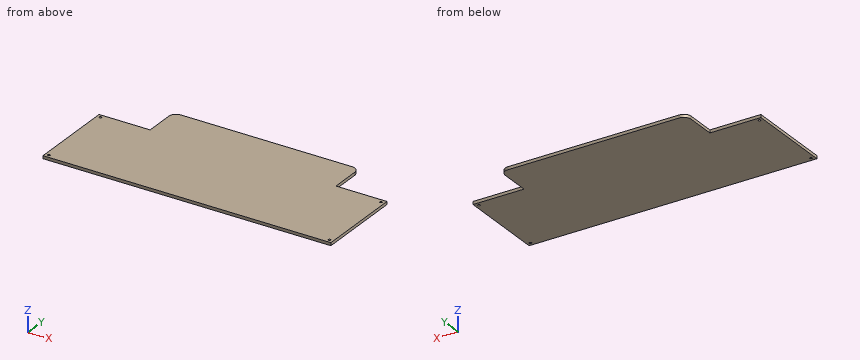
from build123d import *

# Parameters (mm, degrees)
SKETCH_1_R      = 1.6
EXTRUDE_1_DEPTH = 4


with BuildPart() as part:
    # 草图1 → 凸台-拉伸1 (new body)
    with BuildSketch(Plane.XY):
        with BuildLine():
            Line((-197.5, 60), (-127.5, 60))
            Line((-127.5, 60), (-127.5, 100))
            ThreePointArc((-127.5, 100), (-124.571067812, 107.071067812), (-117.5, 110))
            Line((-117.5, 110), (117.5, 110))
            ThreePointArc((117.5, 110), (124.571067812, 107.071067812), (127.5, 100))
            Line((127.5, 100), (127.5, 60))
            Line((127.5, 60), (197.5, 60))
            Line((197.5, 60), (197.5, -60))
            Line((197.5, -60), (-197.5, -60))
            Line((-197.5, -60), (-197.5, 60))
        make_face()
        with Locations((-192.5, 55)):
            Circle(SKETCH_1_R, mode=Mode.SUBTRACT)
        with Locations(Location((192.5, 55, 0), (0, 0, 180))):
            Circle(SKETCH_1_R, mode=Mode.SUBTRACT)
        with Locations((192.5, -55)):
            Circle(SKETCH_1_R, mode=Mode.SUBTRACT)
        with Locations(Location((-192.5, -55, 0), (0, 0, 180))):
            Circle(SKETCH_1_R, mode=Mode.SUBTRACT)
    extrude(amount=EXTRUDE_1_DEPTH)


solid = part.part
Build history of the part. All positions in model axes, mm. Round coordinates to 2 decimals unless told otherwise and drop trailing zeros. Write each loop counter-clockwise with the first axis right and the second up, starting at its lowest first coordinate (ties: lowest second). Pieces come first, ordered by that corner, then holes. Notation, with made-up numbers: M -20,59 L 22,59 A10 cw 22,63 Z; hole C -14,73 d5. An arc over 180 degrees is marked long. Use CSV: the item, a comma, the result in double quotes.
1. Saw through at C-C (x = 159.5). Give the cut face in (y, z).
Reply:
outline,"M -60,0 L 60,0 L 60,4 L -60,4 Z"
2. Wall check: probe 1 along Y at (x, z) = (192.5, 2.9); probe 2 along Y at (x, z) = (135, 1.95); probe 3 along X at (y, z) = (95, 0.55). Give the ranges that are in metal, low to high. Write a range as from..to.
Reply:
probe 1,"y = -60..-56.6, -53.4..53.4, 56.6..60"
probe 2,"y = -60..60"
probe 3,"x = -127.5..127.5"
3. Flat gauge pins, fed straight in: pin 1 (3.5 mm diameter, centred on x = -192.5, y = 55, fed in from +Z); pin 2 (2 mm diameter, centred on y = 74, z = 2.5, fed in from -X); pin 3 (2 mm diameter, centred on x = -156, z = 3, fed in from +Y); pin 4 (2 mm diameter, centred on y = 83, z = 1, fed in from +X). Where does each tip first touch, or does it go through?
Reply:
pin 1,"stops at z = 4"
pin 2,"stops at x = -127.5"
pin 3,"stops at y = 60"
pin 4,"stops at x = 127.5"
4. Saw through at A-A (z = 1). Give the cut face in (x, y).
Reply:
outline,"M -197.5,-60 L 197.5,-60 L 197.5,60 L 127.5,60 L 127.5,100 A10 ccw 117.5,110 L -117.5,110 A10 ccw -127.5,100 L -127.5,60 L -197.5,60 Z; hole C -192.5,-55 d3.2; hole C -192.5,55 d3.2; hole C 192.5,-55 d3.2; hole C 192.5,55 d3.2"
5. Saw through at B-B (y = 75.5). Give the cut face in (x, z).
Reply:
outline,"M -127.5,0 L 127.5,0 L 127.5,4 L -127.5,4 Z"
